Build history of the part. All positions in model axes, mm. Face numbers are marked on the shaded views. A direction names the side the tool comes from. Round coordinates to 2 decimals unless told otherwise and drop trailing zeros. Write each loop counter-clockwise with the first axis right and the second up, starting at its lowest first coordinate (ties: lowest second). Pieces come first, ordered by that corner, then holes. Notation, with made-up numbers: M 32.5,47.25 L 74.5,47.25 A9 ccw 74.5,55.25 Z; hole C 43,64 d5. An arc over 180 degrees is marked long. Write item = value, one per line. Start each with the question number.
Q1. Probe L1, parallel to Z at x = -32.5, y = -11.5; L2, parallel to Z at x = -8.5, y = -13. List the from-to ranges inside material, lowest first.
Q2. Band-saw the part on A-A on z = 19.5. Write the cut outline in (x, y).
Q3. Band-saw the part on D-D on y = -4.5. Write the cut outline in (x, z), plus the area to 3 significant figures.
Q4. Drop flat-ended pins along their axis: P1, Ø10, axis at x = -37.5, z = 22.5, coming from the +Y side; P2, Ø4.5, axis at x = -34, y = -11.5, coming from the +Z side; P3, Ø2, axis at y = -15, z = 23, coming from the -X side; P4, Ø8, axis at x = -44, y = -10.5, coming from the +Z side. Give the stop position or say it passes through.
Q5. Tool access for the marked faces 1 and 2: list every direction of +Z, -Z, +X, -X, +Y, -Y with a clear straight run to the whole face (end or side of a thin tool).
Q6. Pull direction Y, two halves, no side cores. Call the marked faces 3, 4 and 5: released by +Y, released by -Y, zero draft, split by the parting line, or undercut.
Q7. Band-saw the part on C-C on x = -39.5. Write the cut outline in (y, z), plus the area to 3 significant figures.
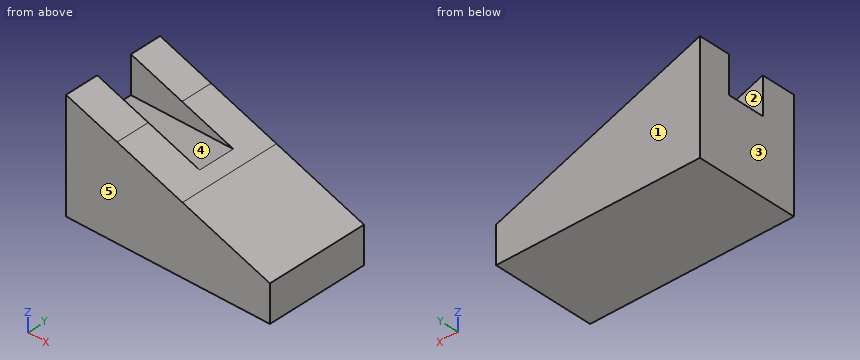
```python
from build123d import *

# Parameters (mm, degrees)
F1_DEPTH = 25.4
F2_W     = 9.1030672193
F2_H     = 9.1277305037
F3_DEPTH = 25.4


with BuildPart() as f1:
    # F0 (on Front) → F1 (new body)
    with BuildSketch(Plane.XZ):
        Polygon((-37.8958209513, 22.6323588295), (-50.5723580718, 27.1732080728), (-50.5723580718, 22.6323588295), align=None)
        Polygon((-37.8958209513, 22.6323588295), (-50.5723580718, 22.6323588295), (-50.5723580718, 9.0577360243), (-21.7006838323, 9.0577360243), (-21.7006838323, 16.8311155222), align=None)
        Polygon((-21.7006838323, 9.0577360243), (-50.5723580718, 9.0577360243), (-50.5723580718, 0), (0, 0), (0, 9.0577360243), align=None)
        Polygon((0, 9.0577360243), (-21.7006838323, 16.8311155222), (-21.7006838323, 9.0577360243), align=None)
    extrude(amount=F1_DEPTH)

    # F2 (on face) → F3 (cut)
    with BuildSketch(Plane(origin=(-50.5723580718, 0, 0), x_dir=(0, -1, 0), z_dir=(-1, 0, 0))):
        with Locations((12.4278347939, 22.6093428209)):
            Rectangle(F2_W, F2_H)
    extrude(amount=-F3_DEPTH, mode=Mode.SUBTRACT)


solid = f1.part
```
Conclusion:
q1.L1 = 0 to 18.05
q1.L2 = 0 to 12.1
q2.outline = M -50.57,-25.4 L -29.15,-25.4 L -29.15,-16.98 L -50.57,-16.98 Z; M -50.57,-7.88 L -29.15,-7.88 L -29.15,0 L -50.57,0 Z
q3.outline = M -50.57,0 L 0,0 L 0,9.06 L -50.57,27.17 Z
q3.area = 916 mm^2
q4.P1 = 0
q4.P2 = 18.05
q4.P3 = through
q4.P4 = 25.9
q5.face_1 = +Z, -Z, +X, -X, +Y
q5.face_2 = +Z, +X, -X
q6.face_3 = zero draft
q6.face_4 = undercut
q6.face_5 = released by -Y
q7.outline = M -25.4,0 L 0,0 L 0,23.21 L -7.88,23.21 L -7.88,18.05 L -16.98,18.05 L -16.98,23.21 L -25.4,23.21 Z
q7.area = 542 mm^2
